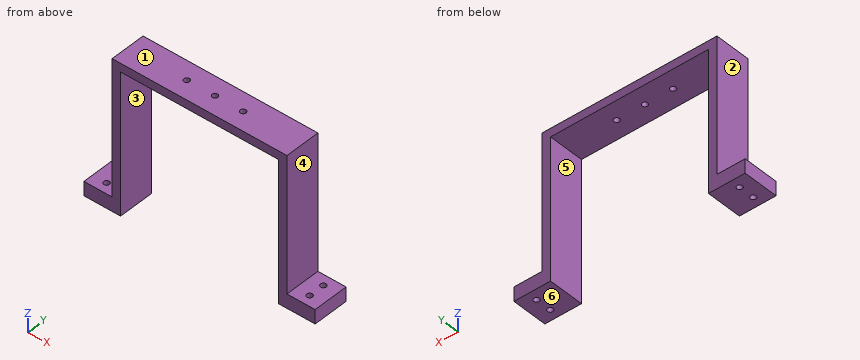
```python
from build123d import *

# Parameters (mm, degrees)
SKETCH1_W           = 62
SKETCH1_H           = 12.6
SKETCH1_R           = 1
BOSS_EXTRUDE1_DEPTH = 3
SKETCH1_14_W        = 3
SKETCH1_14_H        = 12.6
BOSS_EXTRUDE2_DEPTH = 50
SKETCH6_W           = 10
SKETCH6_H           = 12.6
SKETCH6_R           = 1
BOSS_EXTRUDE5_DEPTH = 5


with BuildPart() as part:
    # Sketch1 → Boss-Extrude1 (new body)
    with BuildSketch(Plane.XY):
        with Locations((0, 14.697780108)):
            Rectangle(SKETCH1_W, SKETCH1_H)
        with Locations((0, 14.697780108)):
            Circle(SKETCH1_R, mode=Mode.SUBTRACT)
        with Locations((10, 14.697780108)):
            Circle(SKETCH1_R, mode=Mode.SUBTRACT)
        with Locations((-10, 14.697780108)):
            Circle(SKETCH1_R, mode=Mode.SUBTRACT)
    extrude(amount=BOSS_EXTRUDE1_DEPTH)

    # Sketch1_14 → Boss-Extrude2 (add)
    with BuildSketch(Plane.XY):
        with Locations((-29.5, 14.697780108)):
            Rectangle(SKETCH1_14_W, SKETCH1_14_H)
        with Locations((29.5, 14.697780108)):
            Rectangle(SKETCH1_14_W, SKETCH1_14_H)
    extrude(amount=-BOSS_EXTRUDE2_DEPTH)

    # Sketch6 → Boss-Extrude5 (add)
    with BuildSketch(Plane(origin=(0, 0, -50), x_dir=(-1, 0, 0), z_dir=(0, 0, -1))):
        with Locations((36, 14.697780108)):
            Rectangle(SKETCH6_W, SKETCH6_H)
        with Locations((36, 11.897780108)):
            Circle(SKETCH6_R, mode=Mode.SUBTRACT)
        with Locations((36, 17.497780108)):
            Circle(SKETCH6_R, mode=Mode.SUBTRACT)
        with Locations((-36, 14.697780108)):
            Rectangle(SKETCH6_W, SKETCH6_H)
        with Locations((-36, 11.897780108)):
            Circle(SKETCH6_R, mode=Mode.SUBTRACT)
        with Locations((-36, 17.497780108)):
            Circle(SKETCH6_R, mode=Mode.SUBTRACT)
    extrude(amount=-BOSS_EXTRUDE5_DEPTH)


solid = part.part
```
CAD build for the part. Positions are in the model's coordinates, mm. Face numbers are marked on the shaded views. A direction names the side the tool comes from. Round coordinates to 2 decimals unless told otherwise and drop trailing zeros. Loops run counter-clockwise (first coordinate to the right, second up) from the corner with the lowest first, then second, coordinate; pieces in that order, holes last. Notation, with made-up numbers: M 0,89.25 L 20,89.25 A22 ccw 20,124.25 Z; hole C -26,-34.75 d3. An arc over 180 degrees is marked long. Return JSON: item names as keys, results as strings. Group by question number.
(1) Saw through at D-D, the plane x = 12.5. List the corners of the cut face in (y, z), and give its area (3 significant figures).
(2) Saw through at B-B, the plane z = -42.5. List the corners of the cut face in (x, y), and give its area (3 significant figures).
(3) Saw through at C-C, the plane x = -36. List the corners of the cut face in (y, z), and give its area (3 significant figures).
(4) Wall check: probe 1 along Y at (x, z) = (-36, -47); probe 2 along X at (y, z) = (20, -22); probe 3 along Y at (x, z) = (10, 1). Give the ranges that are in metal, low to high. Write a range as [from, to].
(5) Drop flat-ended pins along their axis: P1, Ø1.8, axis at x = 36, y = 17.5, coming from the -Z side; P2, Ø3, axis at x = -36, y = 11.9, coming from the -Z side; P3, Ø3, axis at x = 36, y = 11.9, coming from the +Z side; P4, Ø5, axis at x = -13, y = 19.5, coming from the -Z side. Give the stop position or say it passes through.
(6) Saw through at A-A, the plane x = 0. List the corners of the cut face in (y, z), and give its area (3 significant figures).
(7) Mould opens along X. For the marked faces 4, 5 and 6 say: +X half, -X half, draft (parallel to the pull), parting line (faces both ways), or undercut.
(8) Tool access for the marked faces 1, 2 and 3: list every direction of +Z, -Z, +X, -X, +Y, -Y with a clear straight run to the whole face (end or side of a thin tool).
Answer list:
{
 "1": {"outline": "M 8.4,0 L 21,0 L 21,3 L 8.4,3 Z", "area": "37.8 mm2"},
 "2": {"outline": "M -31,8.4 L -28,8.4 L -28,21 L -31,21 Z; M 28,8.4 L 31,8.4 L 31,21 L 28,21 Z", "area": "75.6 mm2"},
 "3": {"outline": "M 8.4,-50 L 10.9,-50 L 10.9,-45 L 8.4,-45 Z; M 12.9,-50 L 16.5,-50 L 16.5,-45 L 12.9,-45 Z; M 18.5,-50 L 21,-50 L 21,-45 L 18.5,-45 Z", "area": "43.0 mm2"},
 "4": {"probe 1": "[8.4, 10.9], [12.9, 16.5], [18.5, 21]", "probe 2": "[-31, -28], [28, 31]", "probe 3": "[8.4, 13.7], [15.7, 21]"},
 "5": {"P1": "through", "P2": "z = -50", "P3": "z = -45", "P4": "z = 0"},
 "6": {"outline": "M 8.4,0 L 13.7,0 L 13.7,3 L 8.4,3 Z; M 15.7,0 L 21,0 L 21,3 L 15.7,3 Z", "area": "31.8 mm2"},
 "7": {"face 4": "+X half", "face 5": "undercut", "face 6": "draft"},
 "8": {"face 1": "+Z, +X, -X, +Y, -Y", "face 2": "+Z, -X, +Y, -Y", "face 3": "-Z, +Y, -Y"}
}
